Can you work these out from the model? Positions are in its coordinate system, mm. A direction names the side the tool comes from. Round coordinates to 2 decimals unless told otherwise and drop trailing zeros. Order: outer loops, then holes, each group sorted by start corner. A loop starts at its lowest first (then second) coordinate and runs counter-clockwise, first axis right, second up. Notation, with made-up numbers: M 76.5,89 L 85.5,89 A23 cw 85.5,99 Z; hole C -15,28.25 d1. An arc over 180 degrees is marked long. Answer as a JSON object with one key per item and string values. Group by question number.
from build123d import *

# Parameters (mm, degrees)
F1_DEPTH       = 25
F3_DEPTH       = 10
F5_D           = 8
F5_CBORE_D     = 16
F5_CBORE_DEPTH = 3


with BuildPart() as f1:
    # F0 (on Top) → F1 (new body)
    with BuildSketch(Plane.XY):
        with BuildLine():
            Line((300, 519.615242), (275, 476.313972))
            ThreePointArc((275, 476.313972), (476.313972, 275), (550, 0))
            Line((550, 0), (600, 0))
            ThreePointArc((600, 0), (519.615242, 300), (300, 519.615242))
        make_face()
    extrude(amount=F1_DEPTH)

    # F2 (on face) → F3 (cut)
    with BuildSketch(Plane.XY.offset(25)):
        with BuildLine():
            Line((293.75, 508.789925), (281.25, 487.13929))
            ThreePointArc((281.25, 487.13929), (487.13929, 281.25), (562.5, 0))
            Line((562.5, 0), (587.5, 0))
            ThreePointArc((587.5, 0), (508.789925, 293.75), (293.75, 508.789925))
        make_face()
    extrude(amount=-F3_DEPTH, mode=Mode.SUBTRACT)

    # F5 (through all)
    with Locations(Plane.XY.offset(15)):
        with Locations((497.964607, 287.5), (384.750099, 427.308275), (562.43487, 119.549222)):
            CounterBoreHole(F5_D / 2, F5_CBORE_D / 2, F5_CBORE_DEPTH)


solid = f1.part
Item 1: On a 3-axis mill with a long thin cutter (end or side, diameter ignored), from which of +Z, -Z, +X, -X, +Y, -Y can I reach the whole of each face in a straight line? I mean faces 1 (the face through (287.675, 498.268, 9.547)), 2 (the face through (502, 274, 15)). Say none if no direction works.
Item 2: I need wall thicknesses on line 1 (X direction, y = 40, z = 17.5); line 2 (X direction, y = 93, z = 17.25); line 3 (Y direction, x = 461.5, z = 4.5). Which ranges of each line are inside material? Lowest first, please.
Item 3: Suppose I cut it at A-A, the plane z = 19. Write out the boundary of the cut face in (x, y).
Item 4: Suppose I cut it at B-B, the plane x = 444.5. Write out the boundary of the cut face in (y, z).
Item 5: If we mould it in two halves opening along X, with no side actions, what happens to faces 3 (the face through (492.07, 292.91, 13.52)), 4 (the face through (510.93, 290.01, 20.07)), 5 (the face through (474.29, 278.48, 12.32)), 6 (the face through (485, 280, 0))? For each: +X half, -X half, draft (parallel to the pull), parting line (faces both ways), or undercut.
Item 6: Suppose I cut it at C-C, the plane y = 266.5. Write out the boundary of the cut face in (x, z).
Item 7: I'm going to push flat-ended pins straight in: pin 1 Ø18.5 at (x, y) = (384.75, 427.31) entering from +Z; pin 2 Ø9.5 at (x, y) = (497.96, 287.5) entering from +Z; pin 3 Ø6 at (x, z) = (356, 9) entering from -Y. Where does each tip first touch, or does it pass through?
Computed:
{
 "1": {"face 1": "+Z, -Z, -X, +Y", "face 2": "+Z"},
 "2": {"line 1": "x = 548.54 to 561.08, 586.14 to 598.67", "line 2": "x = 542.08 to 554.76, 580.09 to 592.75", "line 3": "y = 299.2 to 383.43"},
 "3": {"outline": "M 275,476.31 A550 cw 550,0 L 562.5,0 A562.5 ccw 281.25,487.14 Z; M 293.75,508.79 A587.5 cw 587.5,0 L 600,0 A600 ccw 300,519.62 Z"},
 "4": {"outline": "M 323.91,0 L 403.01,0 L 403.01,25 L 384.16,25 L 384.16,15 L 344.71,15 L 344.71,25 L 323.91,25 Z"},
 "5": {"face 3": "undercut", "face 4": "undercut", "face 5": "-X half", "face 6": "draft"},
 "6": {"outline": "M 481.12,0 L 537.57,0 L 537.57,25 L 523.58,25 L 523.58,15 L 495.36,15 L 495.36,25 L 481.12,25 Z"},
 "7": {"pin 1": "stops at z = 15", "pin 2": "stops at z = 12", "pin 3": "stops at y = 416.68"}
}
